For this review, take the finished solid that the model builds, in its own axes (mm). A direction names the side the tool comes from. Coordinates: 2 decimals unless noted, no trailing zeros. Loops run counter-clockwise (first coordinate to the right, second up) from the corner with the lowest first, then second, coordinate; pieces in that order, holes last. Notation, with made-up numbers: M 46,-25.75 L 53,-25.75 A14 cw 53,-16.75 Z; hole C 84,-4.75 d11. An arc over 180 degrees is marked long. Answer as a JSON object with one key per item and string values. Group by question number.
Item 1: Add section B-B (x = 0). State the section outline as (y, z) points.
Item 2: Tool access review of faces 1 (the face through (0, 0, 0)), 2 (the face through (0.78, 34.43, 2.48)): name each direction out of +Z, -Z, +X, -X, +Y, -Y from which nothing blocks a thin tool from reaching the whole face with its end or side.
Item 3: Wall thickness on L1, parallel to Y at x = -2.5, z = 3.25; L2, parallel to X at y = 58.5, z = 0; L3, parallel to X at y = 22, z = -1.75: over which ranges is each line inside the solid? List them lowest first. Write a range as from..to.
Item 4: Insertion check: pin 1 (1 mm diameter, centred on x = 1.5, y = 40, fed in from +Z); pin 2 (1 mm diameter, centred on x = -0.5, y = 17.5, fed in from -Z). Each pin has a flat end and moves straight along its axis. Give the tip position at first contact, or say it passes through.
Item 5: Add section A-A (z = 0). State the section outline as (x, y) points.
from build123d import *

# Parameters (mm, degrees)
SKETCH1_R           = 2.6
BOSS_EXTRUDE1_DEPTH = 69
SKETCH2_R           = 4.25
BOSS_EXTRUDE2_DEPTH = 5
FILLET1_R           = 0.5
CHAMFER1_SIZE       = 0.75
CHAMFER1_SIZE2      = 1.299038106


with BuildPart() as part:
    # Sketch1 → Boss-Extrude1 (new body)
    with BuildSketch(Plane(origin=(0, 0, 0), x_dir=(1, 0, 0), z_dir=(0, 1, 0))):
        with Locations(Location((0, 0, 0), (0, 0, 270))):
            Circle(SKETCH1_R)
    extrude(amount=BOSS_EXTRUDE1_DEPTH)

    # Sketch2 → Boss-Extrude2 (add)
    with BuildSketch(Plane(origin=(0, 69, 0), x_dir=(1, 0, 0), z_dir=(0, 1, 0))):
        with Locations(Location((0, 0, 0), (0, 0, 270))):
            Circle(SKETCH2_R)
    extrude(amount=BOSS_EXTRUDE2_DEPTH)

    # Fillet1
    fillet1_edges = [part.edges().sort_by_distance(p)[0] for p in [
        (0, 69, -2.6),
    ]]
    fillet(fillet1_edges, radius=FILLET1_R)

    # Chamfer1
    chamfer1_edges = [part.edges().sort_by_distance(p)[0] for p in [
        (0, 0, -2.6),
    ]]
    chamfer1_side = [part.faces().sort_by_distance(p)[0] for p in [
        (0, 0, 0),
    ]]
    chamfer(chamfer1_edges, length=CHAMFER1_SIZE, length2=CHAMFER1_SIZE2, reference=chamfer1_side[0])


solid = part.part
From the geometry:
{
 "1": {"outline": "M 0,-1.85 L 1.3,-2.6 L 68.5,-2.6 A0.5 cw 69,-3.1 L 69,-4.25 L 74,-4.25 L 74,4.25 L 69,4.25 L 69,3.1 A0.5 cw 68.5,2.6 L 1.3,2.6 L 0,1.85 Z"},
 "2": {"face 1": "+Z, -Z, +X, -X, -Y", "face 2": "-Y"},
 "3": {"L1": "y = 69..74", "L2": "x = -2.6..2.6", "L3": "x = -1.92..1.92"},
 "4": {"pin 1": "stops at z = 2.4", "pin 2": "stops at z = -2.6"},
 "5": {"outline": "M -4.25,69 L -3.1,69 A0.5 cw -2.6,68.5 L -2.6,1.3 L -1.85,0 L 1.85,0 L 2.6,1.3 L 2.6,68.5 A0.5 cw 3.1,69 L 4.25,69 L 4.25,74 L -4.25,74 Z"}
}
